Part model, mm, in its own coordinate system. A direction names the side the tool comes from. Give positions to 0.01 mm unless a question says otherwise; leave off trailing zeros. Write each loop counter-clockwise with the first axis right and the second up, starting at its lowest first coordinate (ties: lowest second). Pieces come first, ordered by that corner, then holes. Notation, with made-up numbers: (45, -33.75) - (91, -33.75) arc R18 cw to (91, -19.75) - close; hole circle Ø4 at (28, 72.5). An arc over 180 degrees is marked (long way). Answer in a Markdown table with one row per item. Add a question column.
1. Probe line 1 along Y through (x, z) = (1, 0); line 2 along Y through (x, z) = (5.2, 0); line 3 along X through (y, z) = (3.75, 2) (3 decimals). List the from-to ranges inside material, lowest first.
2. Which spindle directions (+Z, -Z, +X, -X, +Y, -Y) get a long thin tool onto all of the face, cutting with end or side? Do faces 1 (the flat face through (3.725, 1.4, 1.4)), 2 (the flat face through (7.5, 6, 2)). Say none if no direction does.
3. Band-saw the part on C-C on x = 6.75. Write the cut outline in (y, z).
4. Band-saw the part on A-A on y = 0. Write the cut outline in (x, z) (3 decimals), plus the area to 3 significant figures.
5. Pull direction Y, two halves, no side cores. Call faces 3 (the cylindrical face through (-1.636, 0.541, -1.717)), 4 (the cylindrical face through (-3.525, -1.978, 2.579)), 5 (the flat face through (0, 0.1, -3.4)): released by +Y, released by -Y, zero draft, split by the parting line, or undercut.
6. Band-saw the part on D-D on z = 5.5. Write the cut outline in (x, y) (3 decimals).
7. Drop flat-ended pins along their axis: pin 1 Ø3 at (x, y) = (-0.5, 6.5) entering from -Z; pin 2 Ø5 at (x, y) = (2, 3) entering from +Z; pin 3 Ø3 at (x, y) = (-0.5, 3.5) entering from -Z. Give the stop position or say it passes through.
```python
from build123d import *

# Parameters (mm, degrees)
SKETCH2_R           = 8
SKETCH2_R_2         = 3.25
BOSS_EXTRUDE1_DEPTH = 7.5
SKETCH3_R           = 6
CUT_EXTRUDE1_DEPTH  = 3.775
SKETCH4_R           = 3.25
SKETCH4_R_2         = 1.8
BOSS_EXTRUDE2_DEPTH = 10.875


with BuildPart() as part:
    # Sketch2 → Boss-Extrude1 (new body)
    with BuildSketch(Plane(origin=(0, 0, 0), x_dir=(0, 0, -1), z_dir=(1, 0, 0))):
        Circle(SKETCH2_R)
        Circle(SKETCH2_R_2, mode=Mode.SUBTRACT)
    extrude(amount=BOSS_EXTRUDE1_DEPTH)

    # Sketch3 → Cut-Extrude1 (cut)
    with BuildSketch(Plane(origin=(7.5, 0, 0), x_dir=(0, 0, -1), z_dir=(1, 0, 0))):
        Circle(SKETCH3_R)
    extrude(amount=-CUT_EXTRUDE1_DEPTH, mode=Mode.SUBTRACT)

    # Sketch4 → Boss-Extrude2 (add)
    with BuildSketch(Plane(origin=(3.725, 0, 0), x_dir=(0, 0, -1), z_dir=(1, 0, 0))):
        Circle(SKETCH4_R)
        Circle(SKETCH4_R_2, mode=Mode.SUBTRACT)
    extrude(amount=-BOSS_EXTRUDE2_DEPTH)


solid = part.part
```
Values:
| question | item | result |
|---|---|---|
| 1 | line 1 | y = -8 to -1.8, 1.8 to 8 |
| 1 | line 2 | y = -8 to -6, 6 to 8 |
| 1 | line 3 | x = 0 to 3.725 |
| 2 | face 1 | +X |
| 2 | face 2 | +Z, -Z, +X, +Y, -Y |
| 3 | outline | circle Ø16 at (0, 0); hole circle Ø12 at (0, 0) |
| 4 | outline | (-7.15, -3.25) - (0, -3.25) - (0, -8) - (7.5, -8) - (7.5, -6) - (3.725, -6) - (3.725, -1.8) - (-7.15, -1.8) - close; (-7.15, 1.8) - (3.725, 1.8) - (3.725, 6) - (7.5, 6) - (7.5, 8) - (0, 8) - (0, 3.25) - (-7.15, 3.25) - close |
| 4 | area | 82.0 mm² |
| 5 | face 3 | undercut |
| 5 | face 4 | split by the parting line |
| 5 | face 5 | zero draft |
| 6 | outline | (0, -5.809) - (7.5, -5.809) - (7.5, -2.398) - (3.725, -2.398) - (3.725, 2.398) - (7.5, 2.398) - (7.5, 5.809) - (0, 5.809) - close |
| 7 | pin 1 | stops at z = -6.18 |
| 7 | pin 2 | stops at z = 7.98 |
| 7 | pin 3 | stops at z = -7.72 |
